Autodesk Inventor part; units mm, degrees
ref_plane "YZ Plane" through (0, 0, 0) normal (1, 0, 0) x (0, 1, 0)
ref_plane "XZ Plane" through (0, 0, 0) normal (0, 1, 0) x (-1, 0, 0)
ref_plane "XY Plane" through (0, 0, 0) normal (0, 0, 1) x (1, 0, 0)
sketch "Skizze1" plane through (0, 0, 0) normal (0, 0, 1) x (1, 0, 0)
  line L0 (-26.25, -95) -> (26.25, -95)
  line L1 (26.25, -95) -> (26.25, 95)
  line L2 (26.25, 95) -> (-26.25, 95)
  line L3 (-26.25, 95) -> (-26.25, -95)
  line L4 (-38.4, 0) -> (46.65, 0)
  line L5 (0, -140.5) -> (0, 178)
  dimension "d0" = 52.5
  dimension "d1" = 190
sketch "Skizze2" plane through (0, 0, 0) normal (0, 1, 0) x (-1, 0, 0)
  line L0 (39, 0) -> (-50.25, 0)
  line L1 (0, -228.1) -> (0, 283.6)
  line L2 (18, 158) -> (18, 210.5)
  line L3 (18, 210.5) -> (-18, 210.5)
  line L4 (-18, 210.5) -> (-18, 158)
  line L5 (-18, 158) -> (-37.5, 158)
  line L6 (-37.5, 158) -> (-37.5, 130)
  line L7 (-37.5, 130) -> (-34.5, 130)
  line L8 (-34.5, 130) -> (-34.5, 155)
  line L9 (-34.5, 155) -> (-15, 155)
  line L10 (-15, 155) -> (-15, 207.5)
  line L11 (-15, 207.5) -> (15, 207.5)
  line L12 (15, 207.5) -> (15, 158)
  line L13 (15, 158) -> (18, 158)
  line L14 (-15, 155) -> (-18, 155)
  line L15 (-18, 155) -> (-18, 130)
  line L16 (-18, 130) -> (-15, 130)
  line L17 (-15, 130) -> (-15, 155)
  point P0 (0, 0)
  dimension "d2" = 3
  dimension "d3" = 3
  dimension "d4" = 3
  dimension "d5" = 3
  dimension "d6" = 3
  dimension "d7" = 30
  dimension "d8" = 19.5
  dimension "d9" = 77.5
  dimension "d10" = 25
  dimension "d11" = 207.5
extrude "Extrusion1" add sketch "Skizze2" along normal mid plane 175
sketch "Skizze3" plane through (0, -87.5, 0) normal (0, -1, 0) x (1, 0, 0)
  line L0 (-18, 210.5) -> (-18, 158)
  line L1 (-18, 158) -> (-15, 158)
  line L2 (-15, 158) -> (-15, 207.5)
  line L3 (-15, 207.5) -> (15, 207.5)
  line L4 (15, 207.5) -> (15, 130)
  line L5 (18, 155) -> (34.5, 155)
  line L6 (34.5, 155) -> (34.5, 130)
  line L7 (34.5, 130) -> (37.5, 130)
  line L8 (37.5, 130) -> (37.5, 158)
  line L9 (37.5, 158) -> (18, 158)
  line L10 (18, 158) -> (18, 210.5)
  line L11 (18, 210.5) -> (-18, 210.5)
  line L12 (34.5, 130) -> (34.5, 155)
  line L13 (34.5, 155) -> (15, 155)
  line L14 (15, 155) -> (15, 130)
  line L15 (15, 130) -> (34.5, 130)
  line L16 (34.5, 130) -> (34.5, 155)
  line L17 (15, 130) -> (18, 130)
  line L18 (18, 130) -> (18, 155)
  line L19 (15, 130) -> (15, 207.5)
extrude "Extrusion2" add sketch "Skizze3" along normal blind 3
sketch "Skizze8" plane through (0, -87.5, 0) normal (0, 1, 0) x (1, 0, 0)
  line L0 (18, -130) -> (18, -155)
  line L1 (18, -155) -> (34.5, -155)
  line L2 (34.5, -155) -> (34.5, -130)
  line L3 (18, -130) -> (34.5, -130)
extrude "Extrusion5" add sketch "Skizze8" along normal blind 11
sketch "Skizze9" plane through (18, 87.5, 158) normal (0, 0, 1) x (1, 0, 0)
  circle A0 centre (9.75, -171) radius 3.75
  line L0 (19.5, 0) -> (19.5, -178) construction
  line L1 (0, 0) -> (19.5, 0)
  line L2 (0, 0) -> (0, -178) construction
  line L3 (19.5, -178) -> (0, -178) construction
  line L4 (16.5, -164) -> (0, -164) construction
  line L5 (0, -164) -> (19.5, -164) construction
  line L6 (19.5, -164) -> (19.5, -178) construction
  line L7 (19.5, -178) -> (0, -178) construction
  line L8 (0, -178) -> (0, -164) construction
  line L9 (0, 0) -> (0, -178)
  line L10 (0, -178) -> (19.5, -164) construction
  line L11 (0, -164) -> (19.5, -178) construction
  dimension "d34" = 7.5
extrude "Extrusion6" cut sketch "Skizze9" against normal through all
chamfer "Fase1" distance 1 angle 45 2 edges at (24, -83.5, 158) (24, -83.5, 130)
sketch "Skizze10" plane through (-18, 87.5, 158) normal (-1, 0, 0) x (0, 0, 1)
  line L0 (0, 0) -> (52.5, 0)
  line L1 (52.5, -178) -> (52.5, 0)
  line L2 (0, 0) -> (52.5, 0)
  line L3 (0, 0) -> (0, -178)
  line L4 (52.5, -178) -> (0, -178)
  line L5 (0, 0) -> (14, 0)
  line L6 (14, 0) -> (14, -14)
  line L7 (14, -14) -> (0, -14)
  line L8 (0, -14) -> (0, 0)
  dimension "d40" = 14
  dimension "d41" = 14
extrude "Extrusion7" add sketch "Skizze10" along normal blind 14 contours L0 L6 L7 L3
fillet "Rundung2" radius 16 1 edges at (-18, 73.5, 165)
fillet "Rundung2" radius 4 1 edges at (-32, 73.5, 165)
fillet "Rundung2" radius 4 1 edges at (-32, 87.5, 165)
sketch "Skizze11" plane through (-32, 87.5, 172) normal (0, 0, 1) x (1, 0, 0)
  circle A0 centre (7, -7) radius 7
  arc A1 (0, -10.7957) -> (2.8, -14.6115) centre (4, -10.7957) ccw
  arc A2 (14, -29.8745) -> (2.8, -14.6115) centre (-2, -29.8745) ccw
  line L0 (14, 0) -> (14, -29.8745)
  line L1 (14, 0) -> (4, 0)
  line L2 (0, -10.7957) -> (0, -4)
  line L3 (14, 0) -> (4, 0)
  line L4 (0, -10.7957) -> (0, -4)
  circle A3 centre (7, -7) radius 3.75
  arc A4 (4, 0) -> (0, -4) centre (4, -4) ccw
  point P0 (0, 0)
  dimension "d46" = 7
  dimension "d47" = 7.5
extrude "Extrusion8" cut sketch "Skizze11" against normal through all contours A3
sketch "Skizze4" plane through (34.5, 87.5, 130) normal (-1, 0, 0) x (0, 0, 1)
  line L0 (25, 0) -> (25, -175)
  line L1 (25, -175) -> (-285, -175)
  line L2 (-285, -175) -> (-285, 45)
  line L3 (-285, 45) -> (25, 45)
  line L4 (25, 45) -> (25, -175)
  dimension "d16" = 310
  dimension "d17" = 220
sketch "Skizze5" plane through (-18, 87.5, 158) normal (-1, 0, 0) x (0, 0, 1)
  line L0 (6, -5) -> (46.5, -5) construction
  line L1 (6, -2.75) -> (46.5, -2.75)
  line L2 (46.5, -7.25) -> (6, -7.25)
  arc A0 (6, -2.75) -> (6, -7.25) centre (6, -5) ccw
  arc A1 (46.5, -7.25) -> (46.5, -2.75) centre (46.5, -5) ccw
  line L3 (-313, 45) -> (-3, 45)
  line L4 (0, 0) -> (0, -178)
  line L5 (52.5, -178) -> (52.5, 0)
  point P0 (26.25, -5)
  dimension "d18" = 4.5
  dimension "d19" = 50
  dimension "d20" = 6
  dimension "d21" = 6
extrude "Extrusion3" [suppressed]
pattern_linear "Rechteckige Anordnung1" [suppressed]
sketch "Skizze13" plane through (0, 87.5, 0) normal (0, 1, 0) x (1, 0, 0)
  line L0 (37.5, -158) -> (37.5, -130)
  line L1 (37.5, -158) -> (18, -210.5)
  line L2 (18, -210.5) -> (15.1877, -209.4554)
  line L3 (15.1877, -209.4554) -> (34.6877, -156.9554)
  line L4 (34.6877, -156.9554) -> (37.5, -158)
  line L5 (18, -210.5) -> (18, -158)
  line L6 (15, -130) -> (15, -207.5)
  dimension "d51" = 3
  dimension "d52" = 3
extrude "Extrusion9" add sketch "Skizze13" against normal blind 160
fillet "Rundung3" radius 7 2 edges at (34.2997, 7.5, 158) (18, -1.5, 158)
sketch "Skizze14" plane through (0, -90.5, 0) normal (0, -1, 0) x (1, 0, 0)
  line L0 (18, 201.8839) -> (18, 165)
  line L1 (37.5013, 157.9968) -> (18, 157.9968)
  line L2 (18, 157.9968) -> (18, 175.3621)
  line L3 (18, 175.3621) -> (37.5013, 175.3621)
  line L4 (37.5013, 175.3621) -> (37.5013, 157.9968)
extrude "Extrusion10" cut sketch "Skizze14" against normal up to surface (18 mm away)
equation "\"d0\" = -0.5 * BreiteTablet + 0.5 * BreitePanel"
equation "\"d2\" = Materialstaerke"
equation "\"d3\" = d2"
equation "\"d4\" = d3"
equation "\"d5\" = d2"
equation "\"d6\" = d5"
equation "\"d7\" = DickePanel"
equation "\"d8\" = DickeTablet + Materialstaerke"
equation "\"d9\" = 0.5 * BreitePanel - 0.5 * BreiteTablet + BreiteRahmenTabletScreen"
equation "\"d10\" = BreiteRahmenTabletScreen"
equation "\"d11\" = 0.5 * BreitePanel"
equation "\"d14\" = Materialstaerke"
equation "\"d41\" = d40"
equation "\"d16\" = BreiteTablet"
equation "\"d17\" = HöheTablet"
equation "\"d18\" = DurchmesserLoch"
equation "\"d19\" = VersatzSchraubeOberkanteTB"
equation "\"d20\" = 2 * Materialstaerke"
equation "\"d21\" = 2 * Materialstaerke"
equation "\"d22\" = Materialstaerke"
equation "\"d26\" = AbstandLochbild"
equation "\"d52\" = d51"
equation "\"BreiteTablet\" = 310"
equation "\"HöheTablet\" = 220"
equation "\"DickeTablet\" = 16.5"
equation "\"BreitePanel\" = 415"
equation "\"DickePanel\" = 30"
equation "\"AbstandLochbild\" = 150"
equation "\"DurchmesserLoch\" = 4.5"
equation "\"VersatzSchraubeOberkanteTB\" = 50"
equation "\"Materialstaerke\" = 3"
equation "\"BreiteRahmenTabletScreen\" = 25"
properties part number "AufnahmeLinks"
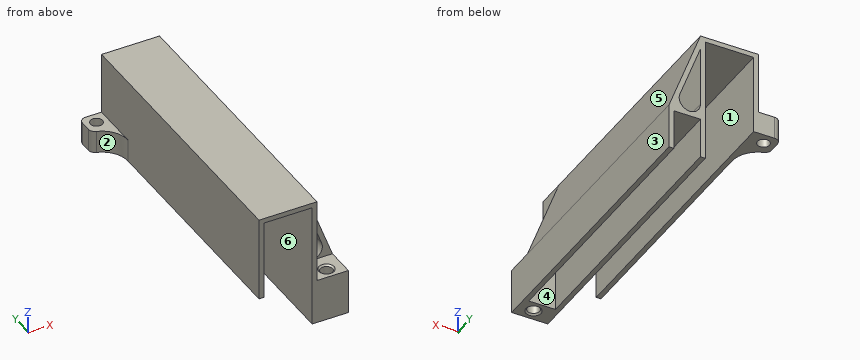
Work out the finished part from the listing and answer in its coordinate system (mm). Face numbers are marked on the shaded views. A direction names the side the tool comes from. Give positions to 0.01 mm unless a question says otherwise; leave off trailing zeros. Loops run counter-clockwise (first coordinate to the right, second up) from the corner with the lowest first, then second, coordinate; pieces in that order, holes last. Notation, with made-up numbers: (-13.5, 66.5) -> (26.5, 66.5) arc R25 ccw to (26.5, 82.5) -> close; hole circle Ø8 at (-26.5, 86.25). An arc over 180 degrees is marked (long way). Use a Markdown table: item, result. Add a question column.
1. Find the intervals of material crossed by probe 1 along X at (y, z) = (-83, 140); probe 2 along X at (y, z) = (-16, 180); probe 3 along X at (y, z) = (31.5, 154), in increasing order.
2. Section C-C on z = 183.5 is taken. Determine the outline of the cut face in (x, y).
3. Flat-ended cylindrical pins translate along their axes: pin 1 Ø1 at (y, z) = (-55.5, 140.5) entering from -X; pin 2 Ø6 at (x, y) = (-25, 80.5) entering from -Z; pin 3 Ø24 at (x, y) = (2.5, -14.5) entering from -Z; pin 4 Ø10 at (x, y) = (-21.5, 46) entering from -Z. Find the tip coordinate at first contact, or state that the pin passes through.
4. Section D-D on y = -83.5 is taken. Determine the outline of the cut face in (x, z).
5. Section B-B on y = -44 is taken. Determine the outline of the cut face in (x, z).
6. Determine the mould class of the marked faces 1, 2 and 3 for opening direction X: released by +X, released by -X, zero draft, split by the parting line, or undercut.
7. Section A-A on y = 80.5 is taken. Determine the outline of the cut face in (x, z), and give its area (3 significant figures).
8. For the marked faces 4, 5 and 6, determine the directions among +Z, -Z, +X, -X, +Y, -Y from which every point of the face is accessible in a straight line to the end or side of a thin tool.
Results below:
| question | item | result |
|---|---|---|
| 1 | probe 1 | x = 15 to 24.03, 31.47 to 37.5 |
| 1 | probe 2 | x = -18 to -15, 15 to 18, 26.13 to 29.33 |
| 1 | probe 3 | x = 15 to 18, 34.5 to 37.5 |
| 2 | outline | (-18, -90.5) -> (-15, -90.5) -> (-15, 87.5) -> (-18, 87.5) -> close; (15, -90.5) -> (18, -90.5) -> (18, 87.5) -> (15, 87.5) -> close; (24.83, -72.5) -> (28.03, -72.5) -> (28.03, 87.5) -> (24.83, 87.5) -> close |
| 3 | pin 1 | stops at x = 15 |
| 3 | pin 2 | passes through |
| 3 | pin 3 | stops at z = 207.5 |
| 3 | pin 4 | stops at z = 158 |
| 4 | outline | (-18, 158) -> (-15, 158) -> (-15, 207.5) -> (15, 207.5) -> (15, 130) -> (23, 130) -> (24, 131) -> (24, 157) -> (23, 158) -> (18, 158) -> (18, 210.5) -> (-18, 210.5) -> close; (31.5, 131) -> (32.5, 130) -> (37.5, 130) -> (37.5, 158) -> (32.5, 158) -> (31.5, 157) -> close |
| 5 | outline | (-18, 158) -> (-15, 158) -> (-15, 207.5) -> (15, 207.5) -> (15, 130) -> (18, 130) -> (18, 155) -> (34.5, 155) -> (34.5, 130) -> (37.5, 130) -> (37.5, 158) -> (18, 210.5) -> (-18, 210.5) -> close; hole (18, 165) arc R7 ccw to (24.62, 158.01) arc R7 ccw to (30.79, 167.44) -> (18, 201.88) -> close |
| 6 | face 1 | undercut |
| 6 | face 2 | released by -X |
| 6 | face 3 | released by +X |
| 7 | outline | (-32, 158) -> (-28.75, 158) -> (-28.75, 172) -> (-32, 172) -> close; (-21.25, 158) -> (-15, 158) -> (-15, 207.5) -> (15, 207.5) -> (15, 130) -> (18, 130) -> (18, 155) -> (34.5, 155) -> (34.5, 130) -> (37.5, 130) -> (37.5, 158) -> (18, 210.5) -> (-18, 210.5) -> (-18, 172) -> (-21.25, 172) -> close; hole (18, 165) arc R7 ccw to (24.62, 158.01) arc R7 ccw to (30.79, 167.44) -> (18, 201.88) -> close |
| 7 | area | 902 mm^2 |
| 8 | face 4 | -Z, +Y |
| 8 | face 5 | +Z, +X, +Y, -Y |
| 8 | face 6 | -Z, +Y, -Y |
